Can you work these out from the drawing? Everything is in mm from the part's minimum corner. A direction names the side the tool comes from. Give positions to 0.01 mm unless a question says otherwise; leave off trailing zeros. Order: outer loops, then holes, each group sorted by start corner. A loop starts at its lowest first (then second) coordinate and runs counter-clockwise, first axis right, second up. Notation, with made-up numbers: (86.25, -23.5) - (110.25, -23.5) arc R18 ccw to (110.25, 7.5) - close; hole circle Ø7 at (4.25, -26.75). An arc over 180 degrees is marked (long way). One line per question, with ' | ' between items.
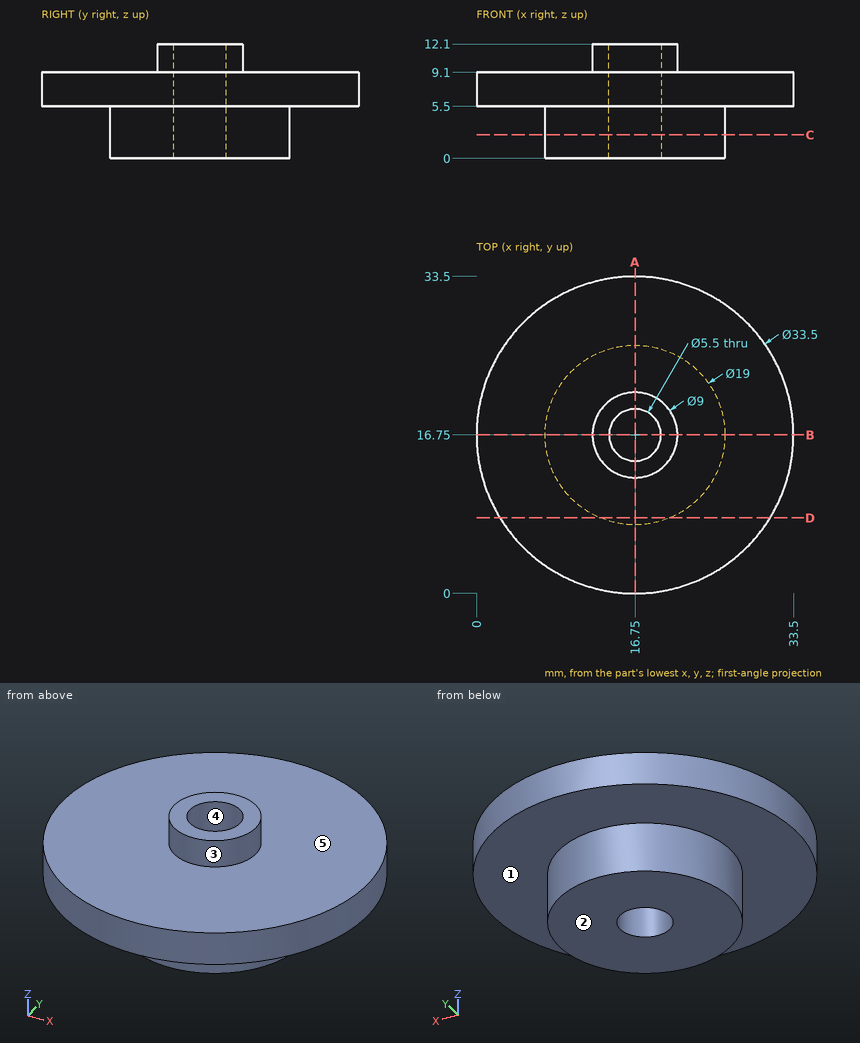
(1) Imagine slicing it at C-C (z = 2.5). List the corners of the cut face in (x, y) for me, and give its area (3 significant figures).
Answer below:
outline: circle Ø19 at (16.75, 16.75); hole circle Ø5.5 at (16.75, 16.75) | area: 260 mm^2
(2) If we mould it in two halves opening along X, with no side actions, what happens to the marked faces 3, 4 and 5? For each: released by +X, released by -X, zero draft, split by the parting line, or undercut.
Answer below:
face 3: split by the parting line | face 4: undercut | face 5: zero draft
(3) If I drill on line 1 (Y direction, x = 16.75, z = 8.25); line 2 (Z direction, x = 16.5, y = 29); line 3 (Z direction, x = 8, y = 19.5), over which ranges is the centre line in solid material (lowest first)?
Answer below:
line 1: 0 to 14, 19.5 to 33.5 | line 2: 5.5 to 9.1 | line 3: 0 to 9.1
(4) Will these pins go through, and if not, where does the flat tip stop? pin 1 (1.5 mm diameter, centred on y = 11.5, z = 9, fed in from +X); pin 2 (5 mm diameter, centred on y = 7.5, z = 6, fed in from -X); pin 3 (1.5 mm diameter, centred on x = 15, z = 5, fed in from +Y).
Answer below:
pin 1: x = 32.88 | pin 2: x = 1.42 | pin 3: y = 33.46
(5) Imagine slicing it at A-A (x = 16.75). List the corners of the cut face in (y, z) for me, and give its area (3 significant figures).
Answer below:
outline: (0, 5.5) - (7.25, 5.5) - (7.25, 0) - (14, 0) - (14, 12.1) - (12.25, 12.1) - (12.25, 9.1) - (0, 9.1) - close; (19.5, 0) - (26.25, 0) - (26.25, 5.5) - (33.5, 5.5) - (33.5, 9.1) - (21.25, 9.1) - (21.25, 12.1) - (19.5, 12.1) - close | area: 186 mm^2
(6) On a 3-axis mill with a long thin cutter (end or side, diameter ignored), from which of +Z, -Z, +X, -X, +Y, -Y can I reach the whole of each face in a straight line? I mean the marked faces 1 and 2. Say none if no direction works.
Answer below:
face 1: -Z | face 2: -Z, +X, -X, +Y, -Y
(7) Imagine slicing it at D-D (y = 8). List the corners of the cut face in (x, z) for me.
Answer below:
outline: (2.47, 5.5) - (13.05, 5.5) - (13.05, 0) - (20.45, 0) - (20.45, 5.5) - (31.03, 5.5) - (31.03, 9.1) - (2.47, 9.1) - close
